Check sheet for the modelled part. Datum: model origin and axes. Units: mm. Round coordinates to 2 decimals unless told otherwise and drop trailing zeros. Order: outer loops, then holes, each group sorted by start corner. A loop starts at its lowest first (then second) coordinate and runs counter-clockwise, first axis right, second up.
(1) Sectioned sample at C-C, the plane x = -70.5. Enter the section's corners in (y, z), and give its area (3 significant figures).
(2) Sectioned sample at A-A, the plane z = 2. Enter the section's corners in (x, y).
(3) Sectioned sample at B-B, the plane y = 100. Enter the section's corners in (x, z), and give its area (3 significant figures).
(4) Thickness scan on probe 1 along X at (y, z) = (-23.5, 2.4); probe 2 along Y at (x, z) = (-50.5, 1.4); probe 3 along X at (y, z) = (-24, 0.7). Record the ranges inside material, lowest first.
(5) Depth check by flat-ended pin: pin 1 (1 mm diameter, centred on x = -61, z = 1.5, fed in from +Y). Enter the tip coordinate at first touch or a pass-through.
```python
from build123d import *

# Parameters (mm, degrees)
BOSS_EXTRU_1_DEPTH      = 3
ESQUISSE2_R             = 1
ENL_V_MAT_EXTRU_1_DEPTH = 3


with BuildPart() as part:
    # Esquisse1 → Boss.-Extru.1 (new body)
    with BuildSketch(Plane.XY):
        with BuildLine():
            Line((33.50283922, 141.076432349), (21.213203436, 128.786796564))
            Line((21.213203436, 128.786796564), (-128.786796564, -21.213203436))
            Line((-128.786796564, -21.213203436), (-141.076432349, -33.50283922))
            ThreePointArc((-141.076432349, -33.50283922), (-142.348197514, -27.604178387), (-143.373440746, -21.657711993))
            Line((-143.373440746, -21.657711993), (-135.857864376, -14.142135624))
            Line((-135.857864376, -14.142135624), (14.142135624, 135.857864376))
            Line((14.142135624, 135.857864376), (21.657711993, 143.373440746))
            ThreePointArc((21.657711993, 143.373440746), (27.604178387, 142.348197514), (33.50283922, 141.076432349))
        make_face()
    extrude(amount=BOSS_EXTRU_1_DEPTH)

    # Esquisse2 → Enlèv. mat.-Extru.1 (cut)
    with BuildSketch(Plane.XY.offset(3)):
        with Locations((6.317279836, 120.961940777)):
            Circle(ESQUISSE2_R)
        with Locations((-120.961940777, -6.317279836)):
            Circle(ESQUISSE2_R)
        with Locations((23.641395976, 138.286056916)):
            Circle(ESQUISSE2_R)
        with Locations((-138.286056916, -23.641395976)):
            Circle(ESQUISSE2_R)
    extrude(amount=-ENL_V_MAT_EXTRU_1_DEPTH, mode=Mode.SUBTRACT)


solid = part.part
```
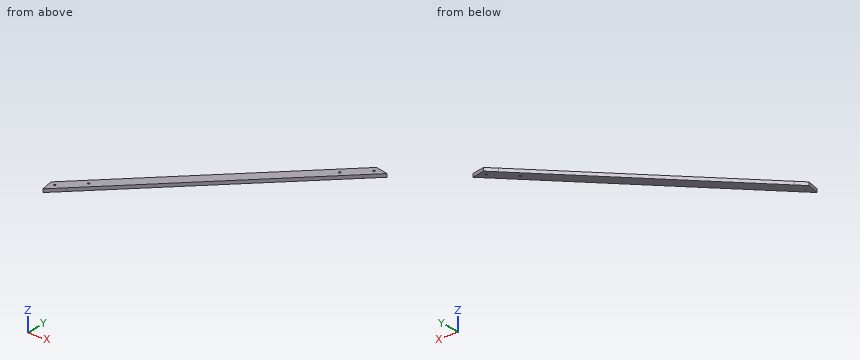
Derived:
1. outline: (37.07, 0) - (51.22, 0) - (51.22, 3) - (37.07, 3) - close
1. area: 42.4 mm2
2. outline: (-143.37, -21.66) arc R145 ccw to (-141.08, -33.5) - (33.5, 141.08) arc R145 ccw to (21.66, 143.37) - close; hole circle Ø2 at (-138.29, -23.64); hole circle Ø2 at (-120.96, -6.32); hole circle Ø2 at (6.32, 120.96); hole circle Ø2 at (23.64, 138.29)
3. outline: (-21.72, 0) - (-7.57, 0) - (-7.57, 3) - (-21.72, 3) - close
3. area: 42.4 mm2
4. probe 1: x = -143.08 to -139.28, -137.3 to -131.07
4. probe 2: y = 57.07 to 71.22
4. probe 3: x = -143 to -139.22, -137.35 to -131.57
5. pin 1: stops at y = 61.22
